Read the model definition and answer for the solid it produces. Units are mm, in the model's axes. A direction names the side the tool comes from. Coordinates: 2 decimals unless noted, no trailing zeros. Loops run counter-clockwise (first coordinate to the right, second up) from the corner with the lowest first, then second, coordinate; pieces in that order, holes last.
Q1. Flat-ended cylindrical pins translate along their axes: P1, Ø4, axis at y = -12, z = 1.5, coming from the -X side; P2, Ø1.7, axis at y = -29, z = 11.5, coming from the -X side; P3, Ø1, axis at x = -20.5, z = 9.5, coming from the -Y side. Find the tip coordinate at first contact, or state that the pin passes through.
Q2. Straight lines are drawn through the part: line 1 (X direction, y = 19.5, z = 1); line 2 (Y direction, x = 0, z = 5); line 3 (Y direction, x = -24.5, z = 7.5). For each, find the intervals that lie inside material, in ascending order.
Q3. Which of the six approach directions +Z, -Z, +X, -X, +Y, -Y give full straight-line access (tool end or side, diameter ignored) to faces 4 (the face through (24.55, -14.62, 11.76)), 5 (the face through (-25.13, -14.07, 10.57)), 6 (the face through (24.67, 21.95, 6.26))?
Q4. Section B-B (z = 5.5) is taken. Give the vertices of the cut face in (x, y), then the cut area to 3 significant figures.
Q5. Section A-A (y = 0) is taken. Give the vertices of the cut face in (x, z) (3 decimals).
Q6. The mould has two halves that part along Y. Classify faces 1 (the face through (24.55, -14.62, 0.94)), 2 (the face through (-28.5, 16.68, 6.26)), 3 (the face through (7, -28, 12.7)): pulls with the +Y half, pulls with the -Y half, needs draft (parallel to the pull), parting line crosses it, or undercut.
Q7. Section C-C (x = 0) is taken. Give the vertices of the cut face in (y, z) (3 decimals), then the cut area to 3 significant figures.
from build123d import *

# Parameters (mm, degrees)
F0_R     = 30.48
F1_DEPTH = 12.7
F2_R     = 30.48
F2_R_2   = 28.575
F3_DEPTH = 3.175
F4_R     = 30.48
F4_R_2   = 28.575
F5_DEPTH = 3.175
F7_DEPTH = 25.4
F8_SIZE  = 1.27


with BuildPart() as f1:
    # F0 (on Top) → F1 (new body)
    with BuildSketch(Plane.XY):
        Polygon((23.1924833864, -25.8367432489), (33.9495698503, -7.2701646691), (31.7390745349, 14.0733697105), (17.4053315185, 30.0413551969), (-3.5766565524, 34.5345640662), (-23.1924833864, 25.8367432489), (-33.9495698503, 7.2701646691), (-31.7390745349, -14.0733697105), (-17.4053315185, -30.0413551969), (3.5766565524, -34.5345640662), align=None)
        Circle(F0_R, mode=Mode.SUBTRACT)
    extrude(amount=F1_DEPTH)

    # F2 (on Top) → F3 (join)
    with BuildSketch(Plane.XY):
        Circle(F2_R)
        Circle(F2_R_2, mode=Mode.SUBTRACT)
    extrude(amount=F3_DEPTH)

    # F4 (on face) → F5 (join)
    with BuildSketch(Plane.XY.offset(12.7)):
        Circle(F4_R)
        Circle(F4_R_2, mode=Mode.SUBTRACT)
    extrude(amount=-F5_DEPTH)

    # F6 (on face) → F7 (cut)
    with BuildSketch(Plane.XY.offset(12.7)):
        with BuildLine():
            ThreePointArc((-25.9621653925, 11.9371936874), (-24.7502578404, 14.2812941233), (-23.3272754336, 16.5036009964))
            Line((-23.3272754336, 16.5036009964), (-24.6366906869, 17.2595922453))
            Line((-24.6366906869, 17.2595922453), (-27.2727255434, 12.6938459433))
            Line((-27.2727255434, 12.6938459433), (-25.9621653925, 11.9371936874))
        make_face()
        with BuildLine():
            ThreePointArc((23.3272754336, 16.5036009964), (24.7466759131, 14.2875), (25.9561754336, 11.9502126283))
            Line((25.9561754336, 11.9502126283), (27.2655906869, 12.7062038773))
            Line((27.2655906869, 12.7062038773), (24.6366906869, 17.2595922453))
            Line((24.6366906869, 17.2595922453), (23.3272754336, 16.5036009964))
        make_face()
        with BuildLine():
            Line((2.6289, -29.9657961227), (2.6289, -28.4538136247))
            ThreePointArc((2.6289, -28.4538136247), (0, -28.575), (-2.6289, -28.4538136247))
            Line((-2.6289, -28.4538136247), (-2.6289, -29.9657961227))
            Line((-2.6289, -29.9657961227), (2.6289, -29.9657961227))
        make_face()
    extrude(amount=-F7_DEPTH, mode=Mode.SUBTRACT)

    # F8
    f8_edges = [f1.edges().sort_by_distance(p)[0] for p in [
        (-24.743092, -14.293705, 3.175),
        (24.746676, -14.2875, 3.175),
        (-24.743092, -14.293705, 9.525),
        (24.746676, -14.2875, 9.525),
        (0, 28.575, 3.175),
        (0, 28.575, 9.525),
    ]]
    chamfer(f8_edges, length=F8_SIZE)


solid = f1.part
Numbers:
1. P1: stops at x = -32.16
1. P2: stops at x = -19.1
1. P3: stops at y = -27.15
2. line 1: x = -26.86 to -20.89, 20.89 to 26.87
2. line 2: y = -33.77 to -30.48, 30.48 to 33.77
2. line 3: y = -22.14 to -18.13, 18.13 to 23.58
3. face 4: +Z, -Z
3. face 5: none
3. face 6: +Z, -Z, +X, +Y
4. outline: (-33.95, 7.27) - (-31.74, -14.07) - (-17.41, -30.04) - (3.58, -34.53) - (23.19, -25.84) - (33.95, -7.27) - (31.74, 14.07) - (17.41, 30.04) - (-3.58, 34.53) - (-23.19, 25.84) - close; hole circle Ø60.96 at (0, 0)
4. area: 624 mm2
5. outline: (-33.197, 0) - (-28.575, 0) - (-28.575, 1.905) - (-29.845, 3.175) - (-30.48, 3.175) - (-30.48, 9.525) - (-29.845, 9.525) - (-28.575, 10.795) - (-28.575, 12.7) - (-33.197, 12.7) - close; (28.575, 0) - (33.197, 0) - (33.197, 12.7) - (28.575, 12.7) - (28.575, 10.795) - (29.845, 9.525) - (30.48, 9.525) - (30.48, 3.175) - (29.845, 3.175) - (28.575, 1.905) - close
6. face 1: undercut
6. face 2: pulls with the +Y half
6. face 3: needs draft
7. outline: (-33.769, 0) - (-29.966, 0) - (-29.966, 3.175) - (-30.48, 3.175) - (-30.48, 9.525) - (-29.966, 9.525) - (-29.966, 12.7) - (-33.769, 12.7) - close; (28.575, 0) - (33.769, 0) - (33.769, 12.7) - (28.575, 12.7) - (28.575, 10.795) - (29.845, 9.525) - (30.48, 9.525) - (30.48, 3.175) - (29.845, 3.175) - (28.575, 1.905) - close
7. area: 97.3 mm2
